Source: CAD feature listing. Evaluate the final solid. Frame: model axes, mm. A direction names the side the tool comes from. Coordinates: 2 decimals unless noted, no trailing zeros. Loops run counter-clockwise (first coordinate to the right, second up) from the corner with the lowest first, then second, coordinate; pieces in that order, holes last. Notation, with made-up numbers: M -29,-25 L -2,-25 A25 ccw -2,-6 Z; hole C 81.5,56 d9. An arc over 180 degrees is marked long. One line per question, with ' | ' between items. Start each with the question number.
1. Section query D-D, the plane z = 5.25. Output: boundary loops of the cut face in (x, y).
2. Access query for faces 1 (the flat face through (0.32, 6.33, -5.1)), 2 (the flat face through (-0.32, -6.37, -5.06)), 3 (the cylindrical face through (-0.321, 6.896, 5.586)), 4 (the flat face through (-37, -8.89, 0)), 5 (the flat face through (37, -8.89, 0)). Directions: +Z, -Z, +X, -X, +Y, -Y. A direction counts if a zero-diameter tool reaches every point of the face in a straight line with its end or side. Return the directions, or none.
3. Section query A-A, the plane z = -1.5. Output: boundary loops of the cut face in (x, y).
4. Pin query (flat end, axial travel): P1, Ø4, axis at x = 0.5, z = 1.5, coming from the -Y side; P2, Ø2.5, axis at x = 37, z = 0.5, coming from the +Y side; P3, Ø5, axis at y = 3.5, z = -2, coming from the -X side. Return the tip coordinate at first contact, or that it passes through.
5. Section query C-C, the plane y = 3.75. Output: boundary loops of the cut face in (x, z), and give its area (3 significant figures).
6. Mould query, pull axis X, two halves, no side actions, for faces 6 (the flat face through (-30.44, -4.51, 0.09)), 7 (the flat face through (37, 8.89, 0)), 8 (the cylindrical face through (-31.07, -12.68, 0.05)), 9 (the flat face through (0, 7.62, 0)). Classes: pulls with the +X half, pulls with the -X half, needs draft (parallel to the pull), parting line crosses it, or undercut.
7. Ray query, probe 1 along X at (y, z) = (7.5, 5.75); probe 2 along Y at (x, z) = (14, 1.25); probe 3 along Y at (x, z) = (-29, 4.5). Return the intervals inside material, ascending.
8. Section query B-B, the plane x = 15. Output: boundary loops of the cut face in (y, z).
```python
from build123d import *

# Parameters (mm, degrees)
F1_DEPTH = 6.35
F3_DEPTH = 12.701
F6_R     = 2.54
F7_SIZE  = 2.54


with BuildPart() as f1:
    # F0 (on Top) → F1 (new body, symmetric)
    with BuildSketch(Plane.XY):
        with BuildLine():
            Line((21.59, 7.62), (-21.59, 7.62))
            ThreePointArc((-21.59, 7.62), (-44.45, 0), (-21.59, -7.62))
            Line((-21.59, -7.62), (21.59, -7.62))
            ThreePointArc((21.59, -7.62), (44.45, 0), (21.59, 7.62))
        make_face()
    extrude(amount=F1_DEPTH, both=True)

    # F4: F3 across plane


with BuildPart() as f3:
    # F2 (on face) → F3 (new body, through all)
    with BuildSketch(Plane.XY.offset(6.35)):
        Polygon((-43.232644, 8.89), (-48.365288, 0), (-43.232644, -8.89), (-32.967356, -8.89), (-27.834712, 0), (-32.967356, 8.89), align=None)
    extrude(amount=-F3_DEPTH)


with BuildPart() as f1_1:
    add(f1.part)
    add(f3.part.mirror(Plane.YZ), mode=Mode.SUBTRACT)

    # F5: cut F3
    add(f3.part, mode=Mode.SUBTRACT)

    # F6
    f6_edges = [f1_1.edges().sort_by_distance(p)[0] for p in [
        (0, -7.62, 6.35),
        (-30.913065, 12.672393, 6.35),
        (-30.913065, -12.672393, 6.35),
        (30.913065, -12.672393, 6.35),
        (30.913065, 12.672393, 6.35),
        (0, 7.62, 6.35),
    ]]
    fillet(f6_edges, radius=F6_R)

    # F7
    f7_edges = [f1_1.edges().sort_by_distance(p)[0] for p in [
        (-30.913065, 12.672393, -6.35),
        (-30.913065, -12.672393, -6.35),
        (0, -7.62, -6.35),
        (30.913065, -12.672393, -6.35),
        (30.913065, 12.672393, -6.35),
        (0, 7.62, -6.35),
    ]]
    chamfer(f7_edges, length=F7_SIZE)


solid = f1_1.part
```
Taken from the geometry:
1) outline: M -40.18,-8.89 A12.25 ccw -21.82,-7.17 L 21.82,-7.17 A12.25 ccw 40.18,-8.89 L 32.97,-8.89 L 27.83,0 L 32.97,8.89 L 40.18,8.89 A12.25 ccw 21.82,7.17 L -21.82,7.17 A12.25 ccw -40.18,8.89 L -32.97,8.89 L -27.83,0 L -32.97,-8.89 Z
2) face 1: -Z, +Y | face 2: -Z, -Y | face 3: +Z, +Y | face 4: +Z, -Z, -X | face 5: +Z, -Z, +X
3) outline: M -40.82,-8.89 A12.7 ccw -21.59,-7.62 L 21.59,-7.62 A12.7 ccw 40.82,-8.89 L 32.97,-8.89 L 27.83,0 L 32.97,8.89 L 40.82,8.89 A12.7 ccw 21.59,7.62 L -21.59,7.62 A12.7 ccw -40.82,8.89 L -32.97,8.89 L -27.83,0 L -32.97,-8.89 Z
4) P1: y = -7.62 | P2: y = 12.05 | P3: x = -31.3
5) outline: M -30,-6.35 L 30,-6.35 L 30,6.35 L -30,6.35 Z | area: 762 mm^2
6) face 6: pulls with the -X half | face 7: needs draft | face 8: undercut | face 9: undercut
7) probe 1: -32.16 to -22.64, 22.64 to 32.16 | probe 2: -7.62 to 7.62 | probe 3: -12.3 to -2.02, 2.02 to 12.3
8) outline: M -7.62,-3.81 L -5.08,-6.35 L 5.08,-6.35 L 7.62,-3.81 L 7.62,3.81 A2.54 ccw 5.08,6.35 L -5.08,6.35 A2.54 ccw -7.62,3.81 Z
